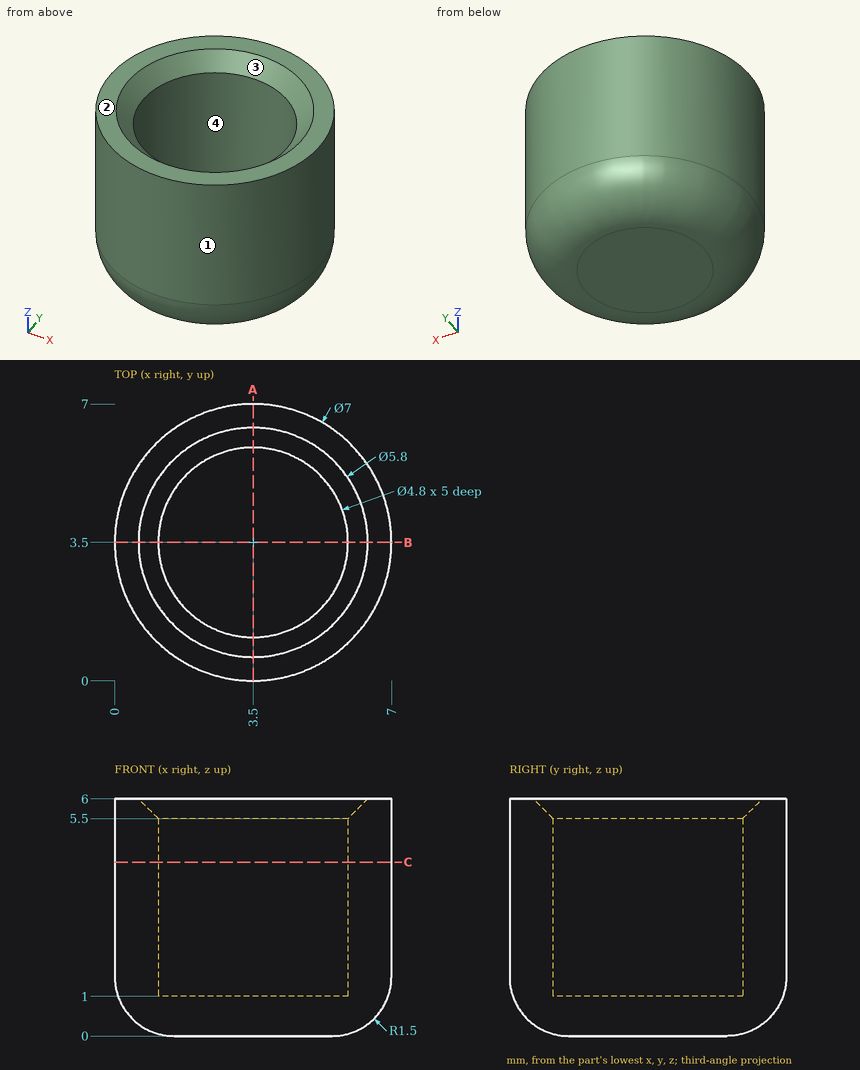
The drawing under review shows one solid part. Ordinate dimensions are in mm from its lowest x, y, z. Give positions to 0.01 mm unless a question says otherwise; leave off trailing zeros. Order: outer loops, then holes, each group sorted by start corner. A loop starts at its lowest first (then second) coordinate and runs counter-clockwise, first axis right, second up. Notation, with made-up numbers: (18, 42.5) - (32, 42.5) arc R23 cw to (32, 73.5) - close; hole circle Ø2 at (55.5, 17). An arc over 180 degrees is marked (long way). Answer as a JSON object with one key per item and string values. Group by question number.
Item 1: Clearance check with flat-ended pins moving along their axes: pin 1 Ø2 at (x, y) = (3, 5) entering from +Z; pin 2 Ø4 at (x, y) = (4, 4) entering from +Z. State where each tip first meets the part, or that it passes through.
Item 2: Take a section at C-C on z = 4.4. Give the boundary of the cut face in (x, y).
Item 3: Wall thickness on line 1 along Y through (x, z) = (3.5, 4.35); line 2 along Y through (x, z) = (5.5, 1.05); line 3 along X through (y, z) = (5.5, 2.1): over which ranges is each line inside the solid? List them lowest first.
Item 4: Draft analysis for pull direction X (two halves, no side actions). For the marked faces 1, 2, 3 and 4, state which applies: pulls with the +X half, pulls with the -X half, needs draft (parallel to the pull), parting line crosses it, or undercut.
Item 5: Take a section at A-A on x = 3.5. Give the boundary of the cut face in (y, z).
Reported:
{
 "1": {"pin 1": "z = 5.68", "pin 2": "z = 5.81"},
 "2": {"outline": "circle Ø7 at (3.5, 3.5); hole circle Ø4.8 at (3.5, 3.5)"},
 "3": {"line 1": "0 to 1.1, 5.9 to 7", "line 2": "0.71 to 2.17, 4.83 to 6.29", "line 3": "0.63 to 2.17, 4.83 to 6.37"},
 "4": {"face 1": "parting line crosses it", "face 2": "needs draft", "face 3": "undercut", "face 4": "undercut"},
 "5": {"outline": "(0, 1.5) arc R1.5 ccw to (1.5, 0) - (5.5, 0) arc R1.5 ccw to (7, 1.5) - (7, 6) - (6.4, 6) - (5.9, 5.5) - (5.9, 1) - (1.1, 1) - (1.1, 5.5) - (0.6, 6) - (0, 6) - close"}
}
